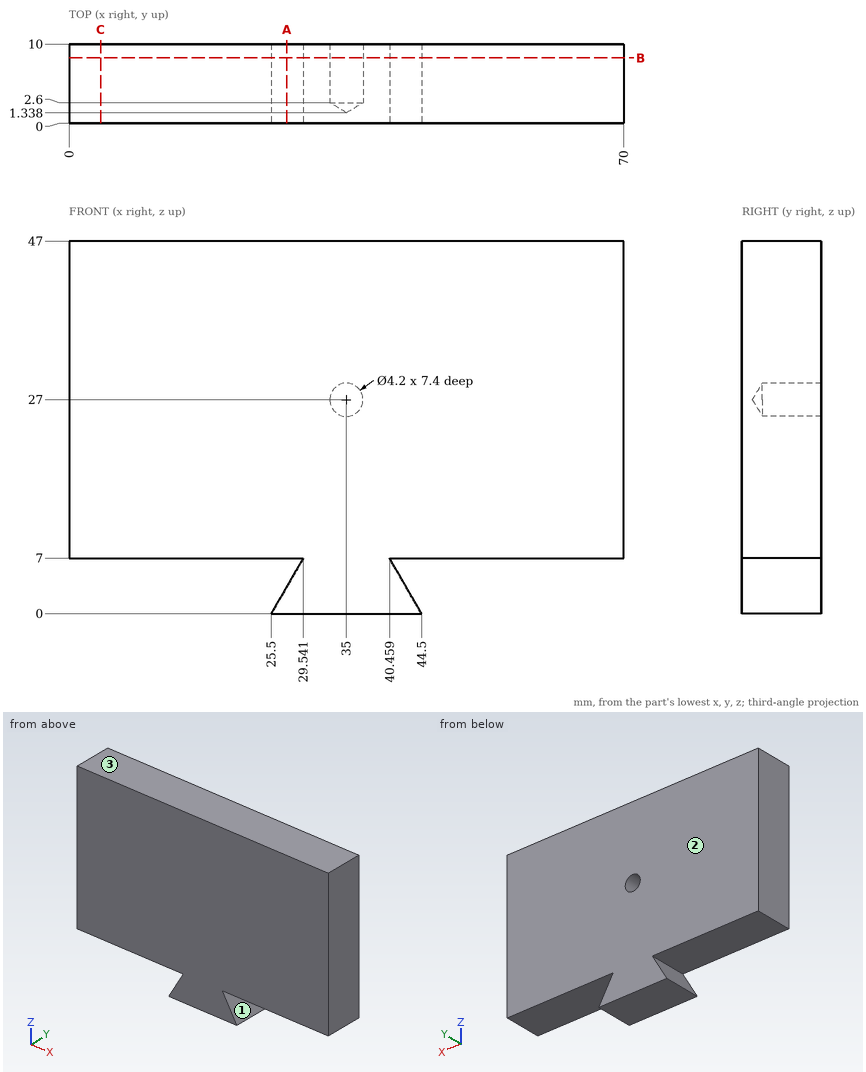
Job drawing, mm, ordinate dimensions from the low corner. One solid piece. Give positions to 0.01 mm unless a question says otherwise; leave off trailing zeros. Loops run counter-clockwise (first coordinate to the right, second up) from the corner with the lowest first, then second, coordinate; pieces in that order, holes last.
Item 1: Slice it at B-B, the plane y = 8.25. List the corners of the cut face in (x, z).
Answers follow:
outline: (0, 7) - (29.54, 7) - (25.5, 0) - (44.5, 0) - (40.46, 7) - (70, 7) - (70, 47) - (0, 47) - close; hole circle Ø4.2 at (35, 27)
Item 2: Slice it at C-C, the plane x = 4. List the corners of the cut face in (y, z), and give its area (3 significant figures).
Answers follow:
outline: (0, 7) - (10, 7) - (10, 47) - (0, 47) - close
area: 400 mm2
Item 3: Flat gauge pin, fed straight in: pin 1 (5 mm diameter, centred on x = 48.5, y = 5.5, fed in from -Z). Where does the tip first touch, or does it go through?
Answers follow:
pin 1: stops at z = 7
Item 4: Slice it at A-A, the plane x = 27.5. List the corners of the cut face in (y, z) (1 decimal), and give its area (3 significant figures).
Answers follow:
outline: (0, 0) - (10, 0) - (10, 3.5) - (0, 3.5) - close; (0, 7) - (10, 7) - (10, 47) - (0, 47) - close
area: 435 mm2
Item 5: Drill centre lines: line 1 (X direction, y = 8, z = 27); line 2 (Z direction, x = 7.5, y = 6.75); line 3 (Z direction, x = 35, y = 6.25). Where is each one in solid material? Low to high.
Answers follow:
line 1: x = 0 to 32.9, 37.1 to 70
line 2: z = 7 to 47
line 3: z = 0 to 24.9, 29.1 to 47
Item 6: Pull direction Z, two halves, no side cores. Call the marked faces 1, 2 and 3: released by +Z, released by -Z, zero draft, split by the parting line, or undercut.
Answers follow:
face 1: undercut
face 2: zero draft
face 3: released by +Z
